Here's how the part is built. I have some questions about the finished solid (model axes, mm). A direction names the side the tool comes from. Round coordinates to 2 decimals unless told otherwise and drop trailing zeros. Write each loop counter-clockwise with the first axis right and the second up, starting at its lowest first coordinate (ties: lowest second). Pieces come first, ordered by that corner, then holes. Notation, with made-up numbers: (27, -19) -> (78, -19) arc R23 cw to (78, 10) -> close; hole circle Ø7 at (64, 65). An arc over 180 degrees is marked (long way). Put each result on its own line as item: value. Start each with the question number.
1. Suppose I cut it at D-D (x = -1.15). Please give me the cut outline in (y, z), then the cut area to 3 significant figures.
2. For pin 1 (1.6 mm diameter, centred on x = -2.5, z = -7.5, fed in from +Y); pin 2 (0.8 mm diameter, centred on x = -2.5, z = -2.5, fed in from +Y); pin 3 (3 mm diameter, centred on y = 6, z = -8, fed in from -X), each with a flat end and sliding along its axis, tell me the tip position at first contact or that it passes through.
3. Which directions (+Z, -Z, +X, -X, +Y, -Y) give clear straight access to the entire face, cutting with the end or side of a thin tool? Please do faces 1 (the face through (-3, 1, -15)), 2 (the face through (-2.5, 2, -2.5)).
4. Suppose I cut it at C-C (z = -12.5). Please give me the cut outline in (x, y), then the cut area to 3 significant figures.
5. We'd pull the mould along X, two halves only. Please class faces 3 (the face through (-2.5, 2, -7.5)), 4 (the face through (-1.694, 4.465, -1.235)), 5 (the face through (-2.5, 2, -5.7)), 6 (the face through (-3.3, 4.5, -13.1)): +X half, -X half, draft (parallel to the pull), parting line (faces both ways), or undercut.
6. Suppose I cut it at A-A (y = 3.75). Please give me the cut outline in (x, z).
7. Suppose I cut it at B-B (x = -2.5). Please give me the cut outline in (y, z), then the cut area to 3 significant figures.
8. I need wall thicknesses on probe 1 along Z at (x, y) = (-2.5, 5.2); probe 2 along X at (y, z) = (3.2, -2.5); probe 3 along Z at (x, y) = (-1.7, 3.5). Which ranges of each line are inside material? Lowest first, please. Write a range as from..to.
Autodesk Inventor part; units mm, degrees
ref_plane "YZ Plane" through (0, 0, 0) normal (1, 0, 0) x (0, 1, 0)
ref_plane "XZ Plane" through (0, 0, 0) normal (0, 1, 0) x (-1, 0, 0)
ref_plane "XY Plane" through (0, 0, 0) normal (0, 0, 1) x (1, 0, 0)
sketch "Sketch1" plane through (0, 0, 0) normal (0, 1, 0) x (-1, 0, 0)
  line L0 (0, 0) -> (5, 0)
  line L1 (5, 0) -> (5, -15)
  line L2 (5, -15) -> (0, -15)
  line L3 (0, -15) -> (0, 0)
  dimension "d0" = 5
  dimension "d1" = 15
extrude "Extrusion1" add sketch "Sketch1" along normal blind 2
sketch "Sketch2" plane through (0, 2, 0) normal (0, 1, 0) x (1, 0, 0)
  line L0 (0, 0) -> (0, 2.5)
  line L1 (0, 2.5) -> (0, 7.5)
  line L2 (0, 7.5) -> (0, 12.5)
  line L3 (0, 2.5) -> (-2.5, 2.5)
  circle A0 centre (-2.5, 2.5) radius 0.5
  circle A1 centre (-2.5, 2.5) radius 1.5
  line L4 (0, 7.5) -> (-2.5, 7.5)
  circle A2 centre (-2.5, 7.5) radius 0.75
  circle A3 centre (-2.5, 7.5) radius 1.5
  line L5 (0, 12.5) -> (-2.5, 12.5)
  circle A4 centre (-2.5, 12.5) radius 1
  circle A5 centre (-2.5, 12.5) radius 1.75
  dimension "d4" = 2.5
  dimension "d5" = 5
  dimension "d6" = 5
  dimension "d7" = 2.5
  dimension "d8" = 1
  dimension "d9" = 3
  dimension "d10" = 2.5
  dimension "d11" = 1.5
  dimension "d12" = 3
  dimension "d13" = 2.5
  dimension "d14" = 2
  dimension "d15" = 3.5
extrude "Extrusion2" add sketch "Sketch2" along normal blind 5
properties part number "HoleSizeTest"
Verdict:
1. outline: (0, -15) -> (2, -15) -> (2, -13.61) -> (7, -13.61) -> (7, -11.39) -> (2, -11.39) -> (2, -8.15) -> (7, -8.15) -> (7, -6.85) -> (2, -6.85) -> (2, -3.15) -> (7, -3.15) -> (7, -1.85) -> (2, -1.85) -> (2, 0) -> (0, 0) -> close
1. area: 54.2 mm^2
2. pin 1: stops at y = 7
2. pin 2: stops at y = 2
2. pin 3: stops at x = -4
3. face 1: -Z, +X, -X, +Y, -Y
3. face 2: +Y
4. outline: (-5, 0) -> (0, 0) -> (0, 2) -> (-0.75, 2) -> (-0.75, 7) -> (-1.5, 7) -> (-1.5, 2) -> (-3.5, 2) -> (-3.5, 7) -> (-4.25, 7) -> (-4.25, 2) -> (-5, 2) -> close
4. area: 17.5 mm^2
5. face 3: undercut
5. face 4: parting line
5. face 5: draft
5. face 6: undercut
6. outline: circle Ø3.5 at (-2.5, -12.5); circle Ø3 at (-2.5, -7.5); circle Ø3 at (-2.5, -2.5); hole circle Ø2 at (-2.5, -12.5); hole circle Ø1.5 at (-2.5, -7.5); hole circle Ø1 at (-2.5, -2.5)
7. outline: (0, -15) -> (2, -15) -> (2, -14.25) -> (7, -14.25) -> (7, -13.5) -> (2, -13.5) -> (2, -11.5) -> (7, -11.5) -> (7, -10.75) -> (2, -10.75) -> (2, -9) -> (7, -9) -> (7, -8.25) -> (2, -8.25) -> (2, -6.75) -> (7, -6.75) -> (7, -6) -> (2, -6) -> (2, -4) -> (7, -4) -> (7, -3) -> (2, -3) -> (2, -2) -> (7, -2) -> (7, -1) -> (2, -1) -> (2, 0) -> (0, 0) -> close
7. area: 55.0 mm^2
8. probe 1: z = -14.25..-13.5, -11.5..-10.75, -9..-8.25, -6.75..-6, -4..-3, -2..-1
8. probe 2: x = -4..-3, -2..-1
8. probe 3: z = -14.06..-13.1, -11.9..-10.94, -8.77..-6.23, -3.77..-1.23
